```python
from build123d import *

# Parameters (mm, degrees)
SKETCH1_R                            = 14.2875
SKETCH1_R_2                          = 3.37312
BOSS_EXTRUDE1_DEPTH                  = 3.175
EDGE_FLANGE1_DEPTH                   = 399.923481586
EDGE_FLANGE2_DEPTH                   = 371.853711622
F_11_32_0_34375_DIAMETER_HOLE4_D     = 8.73125
F_1_4_0_25_DIAMETER_HOLE1_D          = 6.35
F_17_64_0_26563_DIAMETER_HOLE2_D     = 6.747002
F_11_32_0_34375_DIAMETER_HOLE2_D     = 8.73125
F_11_32_0_34375_DIAMETER_HOLE3_D     = 8.73125
F_11_32_0_34375_DIAMETER_HOLE3_DEPTH = 3.175
F_10_0_1935_DIAMETER_HOLE1_D         = 4.9149
CUT_EXTRUDE1_DEPTH                   = 50.8
FILLET1_R                            = 3.175


# Sheet-metal steps are written as plain solids
with BuildPart() as part:
    # Sketch1 → Boss-Extrude1 (new body)
    with BuildSketch(Plane(origin=(0, 0, 0), x_dir=(0, 0, -1), z_dir=(1, 0, 0))):
        with BuildLine():
            Line((397.810445414, 0), (254.102325414, 0))
            ThreePointArc((254.102325414, 0), (249.050931346, 2.092355932), (246.958575414, 7.14375))
            Line((246.958575414, 7.14375), (246.958575414, 69.05625))
            ThreePointArc((246.958575414, 69.05625), (244.866219482, 74.107644068), (239.814825414, 76.2))
            Line((239.814825414, 76.2), (46.139825414, 76.2))
            ThreePointArc((46.139825414, 76.2), (41.088431346, 74.107644068), (38.996075414, 69.05625))
            Line((38.996075414, 69.05625), (38.996075414, 7.14375))
            ThreePointArc((38.996075414, 7.14375), (36.903719482, 2.092355932), (31.852325414, 0))
            Line((31.852325414, 0), (-158.75, 0))
            ThreePointArc((-158.75, 0), (-163.240128061, 1.859871939), (-165.1, 6.35))
            Line((-165.1, 6.35), (-165.1, 81.994446987))
            ThreePointArc((-165.1, 81.994446987), (-165.075836333, 82.547885953), (-165.003529232, 83.097112915))
            Line((-165.003529232, 83.097112915), (-100.43180985, 449.301531106))
            ThreePointArc((-100.43180985, 449.301531106), (-98.981933252, 451.446245541), (-96.4172045, 451.798536022))
            Line((-96.4172045, 451.798536022), (287.551897257, 339.965982534))
            Line((287.551897257, 339.965982534), (347.134178996, 293.415202216))
            ThreePointArc((347.134178996, 293.415202216), (348.525632464, 291.907463008), (349.363704269, 290.034749489))
            Line((349.363704269, 290.034749489), (403.949421055, 83.617862545))
            ThreePointArc((403.949421055, 83.617862545), (404.107468334, 82.812983692), (404.160445414, 81.994446987))
            Line((404.160445414, 81.994446987), (404.160445414, 6.35))
            ThreePointArc((404.160445414, 6.35), (402.300573474, 1.859871939), (397.810445414, 0))
        make_face()
        with Locations((-82.55, 179.578)):
            Circle(SKETCH1_R, mode=Mode.SUBTRACT)
        with Locations((-51.675354011, 354.676818486)):
            Circle(SKETCH1_R_2, mode=Mode.SUBTRACT)
        with Locations((321.610445414, 245.95582)):
            Circle(SKETCH1_R, mode=Mode.SUBTRACT)
        with BuildLine():
            Line((25.362018074, 107.95), (259.432488996, 107.95))
            ThreePointArc((259.432488996, 107.95), (279.55833085, 117.854500987), (283.988391562, 139.843662232))
            Line((283.988391562, 139.843662232), (241.393515847, 300.916964234))
            ThreePointArc((241.393515847, 300.916964234), (235.020226293, 312.158932355), (223.940339151, 318.810005043))
            Line((223.940339151, 318.810005043), (68.8320461, 363.985922583))
            ThreePointArc((68.8320461, 363.985922583), (48.314216085, 361.16759873), (36.715203303, 344.009883255))
            Line((36.715203303, 344.009883255), (0.347901148, 137.760663713))
            ThreePointArc((0.347901148, 137.760663713), (5.904489219, 117.023194714), (25.362018074, 107.95))
        make_face(mode=Mode.SUBTRACT)
    extrude(amount=-BOSS_EXTRUDE1_DEPTH)

    # Edge-Flange1 section (across the edge) → Edge-Flange1 (add)
    with BuildSketch(Plane(origin=(-3.175, 454.846873902, 95.529363767), x_dir=(-3.4914813388431334e-15, -0.9601064189437506, 0.2796348767643397), z_dir=(0, -0.2796348767643397, -0.9601064189437506))):
        with BuildLine():
            Line((-3.175, 3.175), (-3.175, 38.1))
            Line((-3.175, 38.1), (0, 38.1))
            Line((0, 38.1), (0, 3.175))
            ThreePointArc((0, 3.175), (0.92993597, 0.92993597), (3.175, 0))
            Line((3.175, 0), (3.175, -3.175))
            ThreePointArc((3.175, -3.175), (-1.315128061, -1.315128061), (-3.175, 3.175))
        make_face()
    extrude(amount=EDGE_FLANGE1_DEPTH)

    # Edge-Flange2 section (across the edge) → Edge-Flange2 (add)
    with BuildSketch(Plane(origin=(-3.175, 83.648445879, 168.130293847), x_dir=(-3.4914813388431334e-15, -0.17364817766692356, -0.9848077530122092), z_dir=(0, 0.9848077530122092, -0.17364817766692356))):
        with BuildLine():
            Line((-3.175, 3.175), (-3.175, 38.1))
            Line((-3.175, 38.1), (0, 38.1))
            Line((0, 38.1), (0, 3.175))
            ThreePointArc((0, 3.175), (0.92993597, 0.92993597), (3.175, 0))
            Line((3.175, 0), (3.175, -3.175))
            ThreePointArc((3.175, -3.175), (-1.315128061, -1.315128061), (-3.175, 3.175))
        make_face()
    extrude(amount=EDGE_FLANGE2_DEPTH)

    # 11/32 (0.34375) Diameter Hole4 (through all)
    with Locations(Plane(origin=(0, 0, 0), x_dir=(0, 0, -1), z_dir=(1, 0, 0))):
        with Locations((391.478225414, 60.325), (315.278225414, 60.325), (315.278225414, 15.875), (391.478225414, 15.875), (23.178225414, 60.325), (23.178225414, 15.875), (-129.221774586, 15.875), (-129.221774586, 60.325)):
            Hole(F_11_32_0_34375_DIAMETER_HOLE4_D / 2)

    # 1/4 (0.25) Diameter Hole1 (through all)
    with Locations(Plane(origin=(0, 0, 0), x_dir=(0, 0, -1), z_dir=(1, 0, 0))):
        with Locations((353.440683712, 249.779512828), (385.908994874, 127)):
            Hole(F_1_4_0_25_DIAMETER_HOLE1_D / 2)

    # 17/64 (0.26563) Diameter Hole2 (through all)
    with Locations(Plane.ZY.offset(3.175)):
        with Locations((-293.708669101, 320.53990281)):
            Hole(F_17_64_0_26563_DIAMETER_HOLE2_D / 2)

    # 11/32 (0.34375) Diameter Hole2 (through all)
    with Locations(Plane(origin=(0, 396.680507326, -115.53480176), x_dir=(1, 0, 0), z_dir=(3.001434441127967e-15, 0.9601064189437506, -0.27963487676433957))):
        with Locations((-22.225, 136.69059512), (-22.225, -15.70940488), (-22.225, -168.10940488)):
            Hole(F_11_32_0_34375_DIAMETER_HOLE2_D / 2)

    # 11/32 (0.34375) Diameter Hole3
    with Locations(Plane(origin=(0, 31.825615837, 180.492036493), x_dir=(1, 0, 0), z_dir=(3.6503775023836e-15, 0.17364817766692356, 0.9848077530122092))):
        with Locations((-22.225, 391.508974703), (-22.225, 264.508974703), (-22.225, 137.508974703)):
            Hole(F_11_32_0_34375_DIAMETER_HOLE3_D / 2, depth=F_11_32_0_34375_DIAMETER_HOLE3_DEPTH)

    # #10 (0.1935) Diameter Hole1 (through all)
    with Locations(Plane(origin=(0, 0, 0), x_dir=(0, 0, -1), z_dir=(1, 0, 0))):
        with Locations((32.555298074, 377.825), (-14.185781926, 107.95), (314.845818074, 107.95), (262.310998074, 311.15)):
            Hole(F_10_0_1935_DIAMETER_HOLE1_D / 2)

    # Sketch31 → Cut-Extrude1 (cut)
    with BuildSketch(Plane(origin=(0, 52.374163006, -9.23497803), x_dir=(1, 0, 0), z_dir=(0, -0.9848077530122092, 0.17364817766692356))):
        with BuildLine():
            Line((-3.175, 176.926417089), (0, 176.926417089))
            ThreePointArc((0, 176.926417089), (-1.859871939, 181.416545149), (-6.35, 183.276417089))
            Line((-6.35, 183.276417089), (-41.275, 183.276417089))
            Line((-41.275, 183.276417089), (-41.275, 180.101417089))
            Line((-41.275, 180.101417089), (-6.35, 180.101417089))
            ThreePointArc((-6.35, 180.101417089), (-4.10493597, 179.171481119), (-3.175, 176.926417089))
        make_face()
    extrude(amount=-CUT_EXTRUDE1_DEPTH, mode=Mode.SUBTRACT)

    # Fillet1
    fillet1_edges = [part.edges().sort_by_distance(p)[0] for p in [
        (-41.275, 450.128530552, 105.121956774),
        (-41.275, 133.952346214, 160.87234873),
        (-41.275, 456.371042842, 95.0854434),
        (-41.275, 344.538489354, -288.883658358),
    ]]
    fillet(fillet1_edges, radius=FILLET1_R)


solid = part.part
```
Could you check a few things on this model? Use its own coordinates, in mm. A direction names the side the tool comes from. Coordinates: 2 decimals unless noted, no trailing zeros. Write item = value, one per line. Start each with the question number.
(1) I need wall thicknesses on line 1 (X direction, y = 220.5, z = -299.5) (3 decimals); line 2 (Y direction, x = -2.5, z = -216); line 3 (Z direction, x = -0.7, y = 311.15). Which ranges of each line are inside material? Lowest first, please. Write a range as [from, to].
(2) Will these pins go through, and if not, where does the flat tip stop? pin 1 (3 mm diameter, centred on y = 305.5, z = -314.5, fed in from -X) (3 decimals); pin 2 (8 mm diameter, centred on x = -4.5, z = -194.5, fed in from -Y); pin 3 (2 mm diameter, centred on x = -7, z = -148, fed in from +Y).
(3) We'd pull the mould along Y, two halves only. Please class faces 1 (the face through (0, 179, 3)), 2 (the face through (-24.057, 399.713, -93.767)), 3 (the face through (-1.565, 246.584, -307.337)): released by +Y, released by -Y, zero draft, split by the parting line, or undercut.
(4) Which directions (+Z, -Z, +X, -X, +Y, -Y) give clear straight access to the entire face, cutting with the end or side of a thin tool? Please do faces 4 (the face through (-1.565, 341.082, -147.472)), 5 (the face through (-41.275, 290, 133)), 6 (the face through (-4.1, 289.4, 130.9)).
Result set:
q1.line_1 = [-3.175, 0]
q1.line_2 = [76.2, 107.95], [321.12, 366.07]
q1.line_3 = [-324.43, -264.77], [-259.85, -235.95], [-30.92, 127.73]
q2.pin_1 = -3.175
q2.pin_2 = 76.2
q2.pin_3 = 387.52
q3.face_1 = zero draft
q3.face_2 = released by -Y
q3.face_3 = undercut
q4.face_4 = +X, -X
q4.face_5 = +Z, -Z, -X, +Y, -Y
q4.face_6 = -X, -Y
